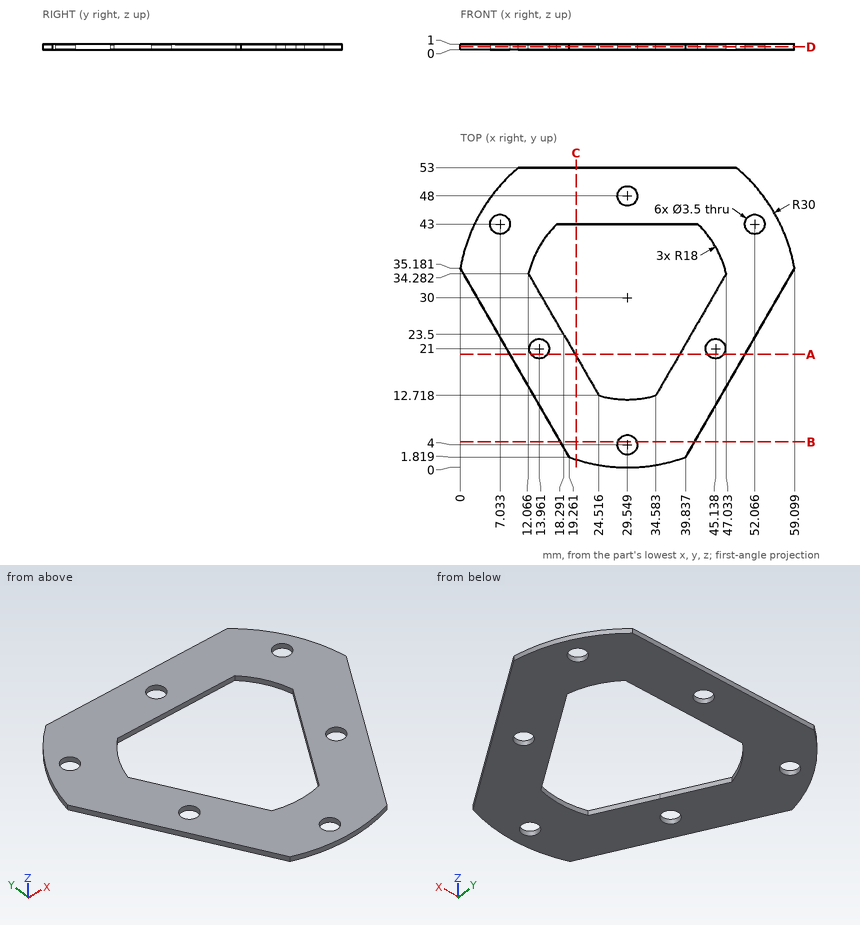
Could you check a few things on this drawing? It's one solid part, dimensions in mm from its lowest x, y, z. Coordinates: 2 decimals unless noted, no trailing zeros. Write each loop counter-clockwise with the first axis right and the second up, starting at its lowest first coordinate (ties: lowest second). Pieces come first, ordered by that corner, then holes. Notation, with made-up numbers: (12.25, 28.5) - (37.25, 28.5) arc R26 ccw to (37.25, 50.5) - close; hole circle Ø7 at (1.25, -34). An arc over 180 degrees is marked (long way). Put each result on its own line as item: value. Start each with the question number.
Q1. Please list where these lines run through material, in increasing order: L1, parallel to X at y = 44, z = 0.65 (1 decimal); L2, parallel to X at y = 25, z = 0.75 (1 decimal); L3, parallel to Y at x = 40.5, z = 0.45 (1 decimal).
Q2. I want a section at C-C on x = 20.5. Write out the boundary of the cut face in (y, z).
Q3. I want a section at A-A on y = 20. Write out the boundary of the cut face in (x, z) (1 decimal).
Q4. I'm going to push a flat-ended pin straight in: P1, Ø0.5, axis at x = 30.5, z = 0.5, coming from the -Y side. Where does the tip first touch, or does it pass through?
Q5. I want a section at B-B on y = 4.5. Write out the boundary of the cut face in (x, z) (1 decimal).
Q6. I want a section at D-D on z = 0.5. Write out the boundary of the cut face in (x, y), plus the area to 3 significant figures.
Checks:
1. L1: 3 to 5.6, 8.5 to 50.6, 53.5 to 56.1
1. L2: 5.9 to 17.4, 41.7 to 53.2
1. L3: 3 to 23, 43 to 53
2. outline: (1.4, 0) - (19.67, 0) - (19.67, 1) - (1.4, 1) - close; (43, 0) - (53, 0) - (53, 1) - (43, 1) - close
3. outline: (8.8, 0) - (12.5, 0) - (12.5, 1) - (8.8, 1) - close; (15.4, 0) - (20.3, 0) - (20.3, 1) - (15.4, 1) - close; (38.8, 0) - (43.7, 0) - (43.7, 1) - (38.8, 1) - close; (46.6, 0) - (50.3, 0) - (50.3, 1) - (46.6, 1) - close
4. P1: y = 0.01
5. outline: (17.7, 0) - (27.9, 0) - (27.9, 1) - (17.7, 1) - close; (31.2, 0) - (41.4, 0) - (41.4, 1) - (31.2, 1) - close
6. outline: (0, 35.18) - (19.26, 1.82) arc R30 ccw to (39.84, 1.82) - (59.1, 35.18) arc R30 ccw to (48.81, 53) - (10.29, 53) arc R30 ccw to start; hole circle Ø3.5 at (7.03, 43); hole (12.07, 34.28) - (18.29, 23.5) - (24.52, 12.72) arc R18 ccw to (34.58, 12.72) - (47.03, 34.28) arc R18 ccw to (42, 43) - (17.1, 43) arc R18 ccw to start; hole circle Ø3.5 at (13.96, 21); hole circle Ø3.5 at (29.55, 4); hole circle Ø3.5 at (29.55, 48); hole circle Ø3.5 at (45.14, 21); hole circle Ø3.5 at (52.07, 43)
6. area: 1,460 mm²
